Autodesk Inventor part; units mm, degrees
ref_plane "YZ Plane" through (0, 0, 0) normal (1, 0, 0) x (0, 1, 0)
ref_plane "XZ Plane" through (0, 0, 0) normal (0, 1, 0) x (-1, 0, 0)
ref_plane "XY Plane" through (0, 0, 0) normal (0, 0, 1) x (1, 0, 0)
sketch "Skizze1" plane through (0, 0, 0) normal (0, 0, 1) x (1, 0, 0)
  circle A0 centre (0, 0) radius 22.5
  dimension "d0" = 45
extrude "Extrusion1" add sketch "Skizze1" along normal mid plane 35
sketch "Skizze2" plane through (0, 0, 17.5) normal (0, 0, 1) x (1, 0, 0)
  circle A0 centre (0, 0) radius 22.5
  circle A1 centre (0, 0) radius 25
  dimension "d3" = 50
extrude "Extrusion2" add sketch "Skizze2" along normal blind 15 contours A0 | A1
sketch "Skizze4" plane through (0, 0, 32.5) normal (0, 0, 1) x (1, 0, 0)
  circle A0 centre (0, 0) radius 25
  circle A1 centre (0, 0) radius 10
  dimension "d6" = 20
extrude "Extrusion3" cut sketch "Skizze4" against normal blind 15 contours A1
chamfer "Fasen1" distance 15 angle 30 1 edges at (-10, 0, 32.5) measured on face at (9.9676, -0.8047, 22.5)
properties part number "Magnethalter"
Input: part model. Units: mm. Frame: model coordinates. A direction names the side the tool comes from. Coordinates: 2 decimals unless noted, no trailing zeros. Loops run counter-clockwise (first coordinate to the right, second up) from the corner with the lowest first, then second, coordinate; pieces in that order, holes last. Notation, with made-up numbers: (-8, -12) -> (27, -12) arc R17 cw to (27, -8) -> close; hole circle Ø8 at (45.25, 45.25). An arc over 180 degrees is marked (long way). One line per item, written item: value.
(1) Ray query, line 1 along Y through (x, z) = (0, 17); line 2 along Y through (x, z) = (0, 17.55); line 3 along X through (y, z) = (-0.5, 21) (3 decimals). Return the intervals inside material, ascending.
Answer below:
line 1: y = -22.5 to 22.5
line 2: y = -25 to -10.03, 10.03 to 25
line 3: x = -24.995 to -12.01, 12.01 to 24.995
(2) Set-up query: faces 4 (the face through (-19, -2, 32.5)), 5 (the face through (-22.34, 3.82, 17.5)). Return all of +Z, -Z, +X, -X, +Y, -Y with unobstructed straight access to the full face (end or side cutting, diameter ignored); none if empty.
Answer below:
face 4: +Z, +X, -X, +Y, -Y
face 5: -Z
(3) Cut plane C-C (z = 2). Output: boundary loops of the cut face in (x, y).
Answer below:
outline: circle Ø45 at (0, 0)
(4) Pin query (flat end, axial travel): pin 1 Ø6 at (x, y) = (3.5, 2) entering from +Z; pin 2 Ø6 at (x, y) = (-6, 14) entering from +Z; pin 3 Ø8 at (x, z) = (6.5, 9.5) entering from +Y. Return the tip coordinate at first contact, or that it passes through.
Answer below:
pin 1: stops at z = 17.5
pin 2: stops at z = 31.76
pin 3: stops at y = 22.36
(5) Draft query along Y for faces 1 (the face through (0, 0, -17.5)), 2 (the face through (10.382, 19.961, -0.245)), 3 (the face through (0, 0, 17.5)). Return one class per face: pulls with the +Y half, pulls with the -Y half, needs draft (parallel to the pull), parting line crosses it, or undercut.
Answer below:
face 1: needs draft
face 2: parting line crosses it
face 3: undercut
